from build123d import *

# Parameters (mm, degrees)
SKETCH2_W                 = 33.655
SKETCH2_H                 = 33.655
BOSS_EXTRUDE1_DEPTH       = 2.38125
CUT_EXTRUDE1_REACH        = 26.27
SKETCH3_W                 = 6.731
SKETCH3_H                 = 6.731
F_4_CLEARANCE_HOLE1_D     = 3.2639
F_4_CLEARANCE_HOLE1_DEPTH = 8.89
F_4_CLEARANCE_HOLE1_TIP   = 0.980574487


with BuildPart() as part:
    # Sketch2 → Boss-Extrude1 (new, symmetric)
    with BuildSketch(Plane.XY):
        Rectangle(SKETCH2_W, SKETCH2_H)
    extrude(amount=BOSS_EXTRUDE1_DEPTH, both=True)

    # Sketch3 → Cut-Extrude1 (cut, up to next)
    with BuildSketch(Plane.XY.offset(2.38125), mode=Mode.PRIVATE) as cut_extrude1_sk1:
        Rectangle(SKETCH3_W, SKETCH3_H)
    cut_extrude1_tool1 = extrude(cut_extrude1_sk1.sketch, amount=-CUT_EXTRUDE1_REACH, mode=Mode.PRIVATE) & part.part
    add(cut_extrude1_tool1.solids().sort_by_distance((0, 0, 2.38125))[0], mode=Mode.SUBTRACT)

    # #4 Clearance Hole1
    with Locations(Plane.XY.offset(2.38125)):
        with Locations((-13.49375, 13.49375), (0, 0), (13.49375, 13.49375), (-13.49375, -13.49375), (13.49375, -13.49375)):
            Hole(F_4_CLEARANCE_HOLE1_D / 2, depth=F_4_CLEARANCE_HOLE1_DEPTH)
            with Locations((0, 0, -(F_4_CLEARANCE_HOLE1_DEPTH + F_4_CLEARANCE_HOLE1_TIP / 2))):  # 118° drill point
                Cone(0, F_4_CLEARANCE_HOLE1_D / 2, F_4_CLEARANCE_HOLE1_TIP, mode=Mode.SUBTRACT)


solid = part.part
Input: part model. Units: mm. Frame: model coordinates. A direction names the side the tool comes from. Round coordinates to 2 decimals unless told otherwise and drop trailing zeros. Order: outer loops, then holes, each group sorted by start corner. A loop starts at its lowest first (then second) coordinate and runs counter-clockwise, first axis right, second up. Notation, with made-up numbers: (6.25, 48.25) - (24.25, 48.25) arc R29 cw to (24.25, 71.25) - close; hole circle Ø6 at (81.5, -20). An arc over 180 degrees is marked (long way). Answer as a JSON object with one key per item and string values. Group by question number.
(1) Draft query along X for faces 3 (the face through (0, 4, 2.381)), 4 (the face through (-15, 12.87, -0.03)), 5 (the face through (3.366, 0, 0)), 6 (the face through (-16.828, 0, 0)). Return one class per face: released by +X, released by -X, zero draft, split by the parting line, or undercut.
(2) Pin query (flat end, axial travel): P1, Ø5, axis at x = -13.49, y = -13.49, coming from the +Z side; P2, Ø2, axis at x = 13.49, y = -13.49, coming from the +Z side. Return the tip coordinate at first contact, or that it passes through.
(3) Material intervals for probe 1 along Y at (x, z) = (13.5, -0.8); probe 2 along X at (y, z) = (-2.5, -1.3), sorted ascending. Write a range as from..to.
(4) Cut plane D-D (z = -0.85). Return loops of the section in (x, y), then the cut area to 3 significant figures.
(5) Cut plane A-A (y = -0.5). Return loops of the section in (x, z), then the cut area to 3 significant figures.
(6) Cut plane C-C (y = -14). Return loops of the section in (x, z), then the cut area to 3 significant figures.
(7) Reachability of faces 1 (the face through (0, 4, -2.381)), 2 (the face through (0, 3.366, 0)) from +Z, -Z, +X, -X, +Y, -Y: full face, straight path, thin tool, end or side. Return the list, or none.
Here are the results:
{
 "1": {"face 3": "zero draft", "face 4": "undercut", "face 5": "undercut", "face 6": "released by -X"},
 "2": {"P1": "stops at z = 2.38", "P2": "passes through"},
 "3": {"probe 1": "y = -16.83..-15.13, -11.86..11.86, 15.13..16.83", "probe 2": "x = -16.83..-3.37, 3.37..16.83"},
 "4": {"outline": "(-16.83, -16.83) - (16.83, -16.83) - (16.83, 16.83) - (-16.83, 16.83) - close; hole circle Ø3.26 at (-13.49, -13.49); hole circle Ø3.26 at (-13.49, 13.49); hole (-3.37, -3.37) - (3.37, -3.37) - (3.37, 3.37) - (-3.37, 3.37) - close; hole circle Ø3.26 at (13.49, -13.49); hole circle Ø3.26 at (13.49, 13.49)", "area": "1,050 mm^2"},
 "5": {"outline": "(-16.83, -2.38) - (-3.37, -2.38) - (-3.37, 2.38) - (-16.83, 2.38) - close; (3.37, -2.38) - (16.83, -2.38) - (16.83, 2.38) - (3.37, 2.38) - close", "area": "128 mm^2"},
 "6": {"outline": "(-16.83, -2.38) - (-15.05, -2.38) - (-15.05, 2.38) - (-16.83, 2.38) - close; (-11.94, -2.38) - (11.94, -2.38) - (11.94, 2.38) - (-11.94, 2.38) - close; (15.05, -2.38) - (16.83, -2.38) - (16.83, 2.38) - (15.05, 2.38) - close", "area": "131 mm^2"},
 "7": {"face 1": "-Z, +X, -X, +Y, -Y", "face 2": "+Z, -Z"}
}
